Geometry check sheet. Reference: the model listing, model coordinates, mm. A direction names the side the tool comes from. Round coordinates to 2 decimals unless told otherwise and drop trailing zeros. Order: outer loops, then holes, each group sorted by start corner. A loop starts at its lowest first (then second) coordinate and runs counter-clockwise, first axis right, second up.
(1) Cross-section at C-C on x = -11.5. Enter the section's corners in (y, z).
(2) Draft check along Y on faces 1 (the face through (0, 77, 3)), 2 (the face through (-1.203, 85.859, 2.958)), 3 (the face through (-39.341, 39, 3)). Enter one of: pulls with the +Y half, pulls with the -Y half, needs draft (parallel to the pull), parting line crosses it, or undercut.
(3) Gauge pin test, flat ends, axial feed: P1, Ø3, axis at x = -19.5, z = 4.5, coming from the -Y side; P2, Ø1.8, axis at y = 80.5, z = 2, coming from the -X side; P3, Ø1.5, axis at y = 20.5, z = 2.5, coming from the -X side; P4, Ø2, axis at x = -23, y = 69.5, coming from the -Z side. Record the tip position at first contact, or that the pin passes through.
(4) Thickness scan on L1, parallel to Y at x = -40, z = 3.3; L2, parallel to Y at x = -30.9, z = 3.9; L3, parallel to X at y = 77.8, z = 3.5. Record the ranges inside material, lowest first.
(5) Cross-section at D-D on z = 1.45. Count the separate pieces of the cut face and the enclosed holes in it, and give its area (3 significant figures).
(6) Cross-section at A-A on y = 77.8. Enter the section's corners in (x, z), and give its area (3 significant figures).
(7) Cross-section at B-B on y = 59. Enter the section's corners in (x, z).
(8) Set-up check for faces 4 (the face through (0, 45, 3)), 5 (the face through (-35.041, 12, 3)), 6 (the face through (-6, 55, 3)), 7 (the face through (-22.244, 7, 3)): record each of +Z, -Z, +X, -X, +Y, -Y from which the full face is reachable in a straight line by a thin tool's end or side.
Autodesk Inventor part; units mm, degrees
ref_plane "YZ Plane" through (0, 0, 0) normal (1, 0, 0) x (0, 1, 0)
ref_plane "XZ Plane" through (0, 0, 0) normal (0, 1, 0) x (-1, 0, 0)
ref_plane "XY Plane" through (0, 0, 0) normal (0, 0, 1) x (1, 0, 0)
sketch "Sketch1" plane through (0, 0, 0) normal (0, 0, 1) x (1, 0, 0)
  arc A0 (0, 83) -> (-4, 87) centre (-4, 83) ccw
  line L0 (-39.2369, 87) -> (-4, 87)
  line L1 (-39.2369, 74.6) -> (-39.2369, 87)
  line L2 (-63, 74.6) -> (-39.2369, 74.6)
  line L3 (-63, 60.5) -> (-63, 74.6)
  line L4 (-39.3408, 60.5) -> (-63, 60.5)
  line L5 (-39.3408, 17.4533) -> (-39.3408, 60.5)
  line L6 (-45.8408, 17.4533) -> (-39.3408, 17.4533)
  line L7 (-45.8408, 13.4533) -> (-45.8408, 17.4533)
  line L8 (-39.8408, 13.4533) -> (-45.8408, 13.4533)
  line L9 (-39.8408, 14.7033) -> (-39.8408, 13.4533)
  line L10 (-38.0408, 14.7033) -> (-39.8408, 14.7033)
  line L11 (-38.0408, 13.4533) -> (-38.0408, 14.7033)
  line L12 (-35.0408, 13.4533) -> (-38.0408, 13.4533)
  line L13 (-35.0408, 10.4533) -> (-35.0408, 13.4533)
  line L14 (-38.0408, 10.4533) -> (-35.0408, 10.4533)
  line L15 (-38.0408, 9.2033) -> (-38.0408, 10.4533)
  line L16 (-39.8408, 9.2033) -> (-38.0408, 9.2033)
  line L17 (-39.8408, 10.4533) -> (-39.8408, 9.2033)
  line L18 (-45.8408, 10.4533) -> (-39.8408, 10.4533)
  line L19 (-45.8408, 5.4533) -> (-45.8408, 10.4533)
  line L20 (-29.0795, 5.4533) -> (-45.8408, 5.4533)
  arc A1 (-23.9205, 5.4533) -> (-29.0795, 5.4533) centre (-26.5, 4.5) ccw
  line L21 (-22.2439, 5.4533) -> (-23.9205, 5.4533)
  line L22 (-22.2439, 8.8497) -> (-22.2439, 5.4533)
  line L23 (-12.4378, 23) -> (-22.2439, 8.8497)
  line L24 (0, 23) -> (-12.4378, 23)
  line L25 (0, 65.75) -> (0, 23)
  line L26 (-2.5, 65.75) -> (0, 65.75)
  arc A2 (-2.5, 71.25) -> (-2.5, 65.75) centre (-2.5, 68.5) ccw
  line L27 (0, 71.25) -> (-2.5, 71.25)
  line L28 (0, 83) -> (0, 71.25)
  line L29 (-27.9, 74.6) -> (-27.9, 81)
  line L30 (-27.9, 81) -> (-16, 81)
  line L31 (-16, 81) -> (-16, 74.6)
  line L32 (-16, 74.6) -> (-27.9, 74.6)
  circle A3 centre (-26.5, 18.5) radius 2.75
  line L33 (-34.7, 60.5) -> (-33.3, 60.5)
  arc A4 (-33.3, 57.5) -> (-33.3, 60.5) centre (-33.3, 59) ccw
  line L34 (-33.3, 57.5) -> (-34.7, 57.5)
  arc A5 (-34.7, 60.5) -> (-34.7, 57.5) centre (-34.7, 59) ccw
  circle A6 centre (-30.9, 77.8) radius 1.5
  circle A7 centre (-3, 59) radius 1.5
  circle A8 centre (-2.5, 82.5) radius 1.5
  circle A9 centre (-60.5, 68.5) radius 1.5
  line L35 (-31, 64) -> (-31, 47)
  line L36 (-24, 64) -> (-31, 64)
  line L37 (-24, 69) -> (-24, 64)
  arc A10 (-22, 71) -> (-24, 69) centre (-22, 69) ccw
  line L38 (-18, 71) -> (-22, 71)
  arc A11 (-16, 69) -> (-18, 71) centre (-18, 69) ccw
  line L39 (-16, 64) -> (-16, 69)
  line L40 (-6, 64) -> (-16, 64)
  line L41 (-6, 47) -> (-6, 64)
  line L42 (-31, 47) -> (-6, 47)
  point P0 (0, 0)
extrude "Extrusion1" add sketch "Sketch1" along normal blind 6
properties part number "yCarTopper"
Found:
1. outline: (23, 0) - (47, 0) - (47, 6) - (23, 6) - close; (64, 0) - (87, 0) - (87, 6) - (64, 6) - close
2. face 1: needs draft
2. face 2: pulls with the +Y half
2. face 3: undercut
3. P1: stops at y = 10.64
3. P2: stops at x = -39.24
3. P3: stops at x = -39.34
3. P4: stops at z = 0
4. L1: y = 5.45 to 10.45, 13.45 to 17.45, 60.5 to 74.6
4. L2: y = 5.45 to 47, 64 to 76.3, 79.3 to 87
4. L3: x = -39.24 to -32.4, -29.4 to -27.9, -16 to 0
5. separate pieces: 1
5. enclosed holes: 8
5. area: 2,610 mm2
6. outline: (-39.24, 0) - (-32.4, 0) - (-32.4, 6) - (-39.24, 6) - close; (-29.4, 0) - (-27.9, 0) - (-27.9, 6) - (-29.4, 6) - close; (-16, 0) - (0, 0) - (0, 6) - (-16, 6) - close
6. area: 146 mm2
7. outline: (-39.34, 0) - (-36.2, 0) - (-36.2, 6) - (-39.34, 6) - close; (-31.8, 0) - (-31, 0) - (-31, 6) - (-31.8, 6) - close; (-6, 0) - (-4.5, 0) - (-4.5, 6) - (-6, 6) - close; (-1.5, 0) - (0, 0) - (0, 6) - (-1.5, 6) - close
8. face 4: +Z, -Z, +X, +Y, -Y
8. face 5: +Z, -Z, -X
8. face 6: +Z, -Z
8. face 7: +Z, -Z, +X, -Y
